Autodesk Inventor part; units mm, degrees
ref_plane "工作平面3" through (0, 0, 16) normal (0, 0, -1) x (-1, 0, 0)
ref_plane "工作平面4" through (0, 0, 2) normal (0, 0, -1) x (-1, 0, 0)
ref_plane "YZ Plane" through (0, 0, 0) normal (1, 0, 0) x (0, 1, 0)
sketch "草圖2" plane through (0, 0, 0) normal (0, 0, 1) x (1, 0, 0)
  circle A0 centre (0, 0) radius 4.5
  dimension "d3" = 9
extrude "擠出2" add sketch "草圖2" along normal blind 40
ref_plane "工作平面3" through (0, 0, 16) normal (0, 0, -1) x (-1, 0, 0)
sketch "草圖5" plane through (0, 0, 16) normal (0, 0, -1) x (-1, 0, 0)
  circle A0 centre (0, 0) radius 5.5
  dimension "d15" = 11
extrude "擠出5" add sketch "草圖5" against normal blind 10
ref_plane "工作平面4" through (0, 0, 2) normal (0, 0, -1) x (-1, 0, 0)
sketch "草圖6" plane through (0, 0, 2) normal (0, 0, -1) x (-1, 0, 0)
  circle A0 centre (0, 0) radius 4
  circle A1 centre (0, 0) radius 4.5
  dimension "d19" = 8
extrude "擠出6" cut sketch "草圖6" against normal blind 1
properties part number "Stage1_carrier_shaft"
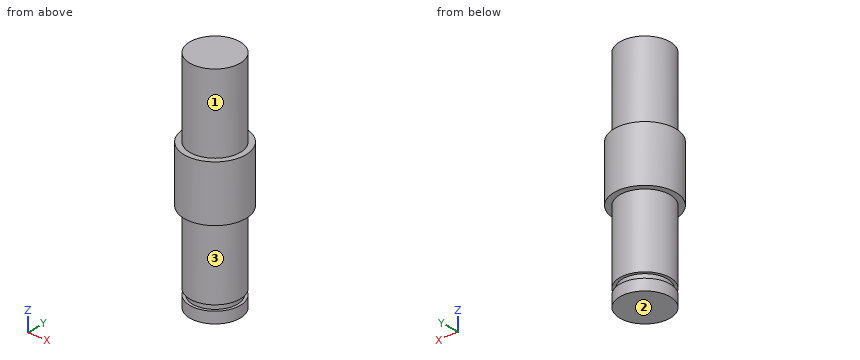
Geometry check sheet. Reference: the model listing, model coordinates, mm. Face numbers are marked on the shaded views. A direction names the side the tool comes from. Coordinates: 2 decimals unless noted, no trailing zeros. Write each loop counter-clockwise with the first axis right and the second up, starting at its lowest first coordinate (ties: lowest second). Pieces come first, ordered by that corner, then holes. Notation, with made-up numbers: M 47.5,-16.75 L 101.5,-16.75 A33 cw 101.5,16.25 Z; hole C 35,-27 d9. An arc over 180 degrees is marked long. Use one line per item in the form item = value. Start each with the question number.
1) Section check A-A on x = 0. Enter the section's corners in (y, z).
2) Thickness scan on probe 1 along Z at (x, y) = (-0.5, -4); probe 2 along Z at (x, y) = (-2.5, 4); probe 3 along Y at (x, z) = (-0.25, 31). Record the ranges inside material, lowest first. Write a range as from..to.
3) Section check D-D on z = 26.5. Enter the section's corners in (x, y), and give its area (3 significant figures).
4) Section check C-C on z = 21. Enter the section's corners in (x, y).
5) Go/stop test with flat-tipped pins: pin 1 Ø4 at (y, z) = (-4, 12.5) entering from -X; pin 2 Ø6 at (x, z) = (-3.5, 14) entering from -Y; pin 3 Ø3 at (y, z) = (2, 15) entering from +X; pin 4 Ø6 at (x, y) = (1.5, 0.5) entering from -Z. Record where each tip stops, or that it passes through.
6) Set-up check for the marked faces 1, 2 and 3: record each of +Z, -Z, +X, -X, +Y, -Y from which the full face is reachable in a straight line by a thin tool's end or side.
Responses:
q1.outline = M -5.5,16 L -4.5,16 L -4.5,3 L -4,3 L -4,2 L -4.5,2 L -4.5,0 L 4.5,0 L 4.5,2 L 4,2 L 4,3 L 4.5,3 L 4.5,16 L 5.5,16 L 5.5,26 L 4.5,26 L 4.5,40 L -4.5,40 L -4.5,26 L -5.5,26 Z
q2.probe_1 = 0..2, 3..40
q2.probe_2 = 16..26
q2.probe_3 = -4.49..4.49
q3.outline = C 0,0 d9
q3.area = 63.6 mm2
q4.outline = C 0,0 d11
q5.pin_1 = -4.03
q5.pin_2 = -5.35
q5.pin_3 = 5.43
q5.pin_4 = 0
q6.face_1 = +Z
q6.face_2 = -Z, +X, -X, +Y, -Y
q6.face_3 = -Z
